```python
from build123d import *

# Parameters (mm, degrees)
F0_R     = 6.35
F1_DEPTH = 2.54


with BuildPart() as f1:
    # F0 (on Front) → F1 (new body)
    with BuildSketch(Plane.XZ):
        with BuildLine():
            Line((-6.8326, 40.622082), (-10.840268, 2.291895))
            Line((-10.840268, 2.291895), (-11.0799, 0))
            ThreePointArc((-11.0799, 0), (0.585254, -11.064433), (11.018073, 1.168874))
            Line((11.018073, 1.168874), (6.8326, 40.622082))
            ThreePointArc((6.8326, 40.622082), (0, 47.454682), (-6.8326, 40.622082))
        make_face()
        Circle(F0_R, mode=Mode.SUBTRACT)
    extrude(amount=F1_DEPTH)


solid = f1.part
```
CAD build for the part. Positions are in the model's coordinates, mm. Round coordinates to 2 decimals unless told otherwise and drop trailing zeros. Loops run counter-clockwise (first coordinate to the right, second up) from the corner with the lowest first, then second, coordinate; pieces in that order, holes last. Notation, with made-up numbers: (89.25, -3) - (120.25, -3) arc R12 ccw to (120.25, 3) - close; hole circle Ø7 at (73.5, 29). An arc over 180 degrees is marked (long way). Return JSON: item names as keys, results as strings. Group by question number.
Q1. Two-plate mould, pull along Z, no slides. Class faces 1 (the face through (8.955, -1.252, 20.619)), 2 (the face through (0, -2.54, 19)), 3 (the face through (-1.38, -1.25, -6.2)): +Z half, -Z half, draft (parallel to the pull), parting line (faces both ways), or undercut.
Q2. Band-saw the part on D-D on x = -9.25. Give the cut face in (y, z).
Q3. Band-saw the part on A-A on x = 0. Give the cut face in (y, z).
Q4. Band-saw the part on C-C on z = 43.5. Give the cut face in (x, y).
Q5. Flat gauge pins, fed straight in: pin 1 Ø1 at (y, z) = (-2, 27.5) entering from +X; pin 2 Ø1.5 at (x, y) = (4, -0.5) entering from +Z; pin 3 Ø1 at (y, z) = (-2, 6.5) entering from -X. Where does each tip first touch, or does it go through?
Q6. Drill centre lines: line 1 along Z through (x, y) = (0, -0.55); line 2 along Z through (x, y) = (5.25, -0.7); line 3 along X through (y, z) = (-0.9, 44.5). Where is each one in solid material? Low to high. Write a range as [from, to].
Q7. Band-saw the part on B-B on y = -1.55. Give the cut face in (x, z).
Solutions:
{
 "1": {"face 1": "+Z half", "face 2": "draft", "face 3": "undercut"},
 "2": {"outline": "(-2.54, -6.1) - (0, -6.1) - (0, 17.5) - (-2.54, 17.5) - close"},
 "3": {"outline": "(-2.54, -11.08) - (0, -11.08) - (0, -6.35) - (-2.54, -6.35) - close; (-2.54, 6.35) - (0, 6.35) - (0, 47.45) - (-2.54, 47.45) - close"},
 "4": {"outline": "(-6.2, -2.54) - (6.2, -2.54) - (6.2, 0) - (-6.2, 0) - close"},
 "5": {"pin 1": "stops at x = 8.28", "pin 2": "stops at z = 46.63", "pin 3": "stops at x = -10.45"},
 "6": {"line 1": "z = [-11.08, -6.35], [6.35, 47.45]", "line 2": "z = [-9.76, -3.57], [3.57, 44.99]", "line 3": "x = [-5.63, 5.63]"},
 "7": {"outline": "(-11.08, 0) arc R11.08 ccw (long way) to (11.02, 1.17) - (6.83, 40.62) arc R6.83 ccw to (-6.83, 40.62) - (-10.84, 2.29) - close; hole circle Ø12.7 at (0, 0)"}
}
